Part model, mm, in its own coordinate system. Round coordinates to 2 decimals unless told otherwise and drop trailing zeros. Loops run counter-clockwise (first coordinate to the right, second up) from the corner with the lowest first, then second, coordinate; pieces in that order, holes last.
(1) Probe probe 1 along Z at (x, y) = (349.5, 16.5); probe 2 along Y at (x, z) = (400.5, -23); probe 3 along Y at (x, z) = (409.5, 2). List the from-to ranges inside material, lowest first.
(2) Cut at C-C on x = 135.5. List the corners of the cut face in (y, z), then the cut area to 3 significant figures.
(3) Flat gauge pins, fed straight in: pin 1 (3 mm diameter, centred on x = 410.5, z = -24.5, fed in from +Y); pin 2 (1.5 mm diameter, centred on x = 381.5, z = 9.5, fed in from +Y); pin 3 (0.7 mm diameter, centred on x = 559.5, z = -19.5, fed in from +Y). Where does each tip first touch, or does it go through?
(4) Cut at B-B on x = 438.5. List the corners of the cut face in (y, z), then the cut area to 3 significant figures.
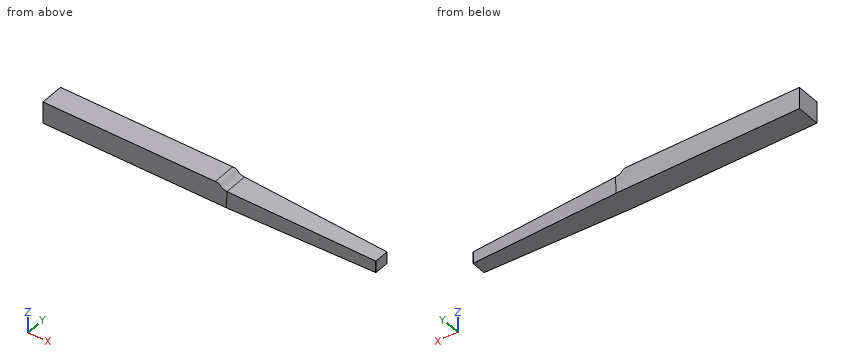
from build123d import *

# Parameters (mm, degrees)
CROQUIS1_W                 = 1120
CROQUIS1_H                 = 73.6
SALIENTE_EXTRUIR2_DEPTH    = 80
CORTAR_EXTRUIR1_DEPTH      = 567.881151565
CORTAR_EXTRUIR1_DEPTH_BACK = 80
CORTAR_EXTRUIR2_DEPTH      = 80
CORTAR_EXTRUIR6_DEPTH      = 80
CROQUIS9_W                 = 1.38989899
CROQUIS9_H                 = 14.75
CORTAR_EXTRUIR7_DEPTH      = 80
CORTAR_EXTRUIR11_DEPTH     = 80
CROQUIS11_W                = 1.38989899
CROQUIS11_H                = 14.75
CORTAR_EXTRUIR12_DEPTH     = 80


with BuildPart() as part:
    # Croquis1 → Saliente-Extruir2 (new body)
    with BuildSketch(Plane(origin=(0, 0, 0), x_dir=(-1, 0, 0), z_dir=(0, 1, 0))):
        Rectangle(CROQUIS1_W, CROQUIS1_H)
    extrude(amount=SALIENTE_EXTRUIR2_DEPTH)

    # Croquis3 → Cortar-Extruir1 (cut, two sides: drawn at the far end of the back side and taken through both)
    with BuildSketch(Plane(origin=(0, 80, 0), x_dir=(-1, 0, 0), z_dir=(0, 1, 0)).offset(-CORTAR_EXTRUIR1_DEPTH_BACK)):
        Polygon((-2813.471365519, -75.102439368), (-560, 3.2), (-65, 20.4), (-65, 36.8), (-560, 36.8), (-2814.831361149, 36.8), (-7324.161069919, -18.003708809), (-7322.801074288, -129.906148176), align=None)
    extrude(amount=CORTAR_EXTRUIR1_DEPTH + CORTAR_EXTRUIR1_DEPTH_BACK, mode=Mode.SUBTRACT)

    # Croquis5 → Cortar-Extruir2 (cut)
    with BuildSketch(Plane(origin=(0, 80, 0), x_dir=(-1, 0, 0), z_dir=(0, 1, 0))):
        with BuildLine():
            Line((-65, 20.4), (-65, 36.8))
            Line((-65, 36.8), (-25, 36.8))
            add(Edge.make_bspline(
                [(-65, 20.4), (-56.784244263, 22.107577244), (-47.818766965, 23.337438109), (-39.843013972, 33.586115732), (-32.987752431, 36.631059032), (-31.175714622, 36.8), (-25, 36.8)],
                knots=[0, 0, 0, 0, 0.422650191, 0.727847648, 0.789397597, 1, 1, 1, 1], degree=3))
        make_face()
    extrude(amount=-CORTAR_EXTRUIR2_DEPTH, mode=Mode.SUBTRACT)

    # Croquis6 → Cortar-Extruir6 (cut)
    with BuildSketch(Plane(origin=(0.786379176, 0, 22.631261168), x_dir=(0.9993968526186474, 0, -0.0347265168990722), z_dir=(0.0347265168990722, 0, 0.9993968526186474))):
        Polygon((64.252374475, 0), (559.551112612, 0), (559.551112612, 14.75), align=None)
    extrude(amount=-CORTAR_EXTRUIR6_DEPTH, mode=Mode.SUBTRACT)

    # Croquis9 → Cortar-Extruir7 (cut)
    with BuildSketch(Plane(origin=(0, 0, -36.8), x_dir=(1, 0, 0), z_dir=(0, 0, -1))):
        with Locations((559.305050505, -7.375)):
            Rectangle(CROQUIS9_W, CROQUIS9_H)
    extrude(amount=-CORTAR_EXTRUIR7_DEPTH, mode=Mode.SUBTRACT)

    # Croquis10 → Cortar-Extruir11 (cut)
    with BuildSketch(Plane(origin=(0.786379176, 0, 22.631261168), x_dir=(0.9993968526186474, 0, -0.0347265168990722), z_dir=(0.0347265168990722, 0, 0.9993968526186474))):
        Polygon((64.252374475, 80), (559.551112612, 65.25), (559.551112612, 80), align=None)
    extrude(amount=-CORTAR_EXTRUIR11_DEPTH, mode=Mode.SUBTRACT)

    # Croquis11 → Cortar-Extruir12 (cut)
    with BuildSketch(Plane(origin=(0, 0, -36.8), x_dir=(1, 0, 0), z_dir=(0, 0, -1))):
        with Locations((559.305050505, -72.625)):
            Rectangle(CROQUIS11_W, CROQUIS11_H)
    extrude(amount=-CORTAR_EXTRUIR12_DEPTH, mode=Mode.SUBTRACT)


solid = part.part
Final values:
1. probe 1: z = -36.8 to 10.51
1. probe 2: y = 10.03 to 69.97
1. probe 3: y = 10.27 to 69.73
2. outline: (2.1, 17.95) - (2.16, -36.8) - (77.84, -36.8) - (77.9, 17.95) - close
2. area: 4,150 mm2
3. pin 1: stops at y = 69.72
3. pin 2: stops at y = 70.59
3. pin 3: stops at y = 65.25
4. outline: (11.13, 7.42) - (11.18, -36.8) - (68.82, -36.8) - (68.87, 7.42) - close
4. area: 2,550 mm2
